```python
from build123d import *

# Parameters (mm, degrees)
SKETCH_1_W                    = 100
SKETCH_1_H                    = 80
EXTRUDE_1_DEPTH               = 19
SKETCH_2_W                    = 72
SKETCH_2_H                    = 92
CUT_EXTRUDE_1_DEPTH           = 17
SKETCH_3_W                    = 36.5
SKETCH_3_H                    = 54.5
EXTRUDE_2_DEPTH               = 17
SKETCH_4_W                    = 31.5
SKETCH_4_H                    = 49.5
CUT_EXTRUDE_2_DEPTH           = 17
HOLE_WIZARD_20_0_20_1_D       = 20
HOLE_WIZARD_20_0_20_1_DEPTH   = 2
HOLE_WIZARD_1_8_1_8_1_D       = 1.8
HOLE_WIZARD_1_8_1_8_2_D       = 1.8
HOLE_WIZARD_1_8_1_8_2_DEPTH   = 4
HOLE_WIZARD_1_8_1_8_3_D       = 1.8
HOLE_WIZARD_1_8_1_8_3_DEPTH   = 4
HOLE_WIZARD_2_35_2_35_1_D     = 2.35
HOLE_WIZARD_2_35_2_35_1_DEPTH = 2.5
HOLE_WIZARD_2_35_2_35_2_D     = 2.35
HOLE_WIZARD_2_35_2_35_2_DEPTH = 2.5
HOLE_WIZARD_2_35_2_35_3_D     = 2.35
HOLE_WIZARD_2_35_2_35_3_DEPTH = 2.5
HOLE_WIZARD_2_35_2_35_4_D     = 2.35
HOLE_WIZARD_2_35_2_35_4_DEPTH = 2.5
SKETCH_22_W                   = 13
SKETCH_22_H                   = 36.5
CUT_EXTRUDE_5_DEPTH           = 10
SKETCH_23_W                   = 80
SKETCH_23_H                   = 22.75
CUT_EXTRUDE_6_DEPTH           = 19
SKETCH_24_W                   = 17
SKETCH_24_H                   = 17.75
EXTRUDE_3_DEPTH               = 4
SKETCH_25_R                   = 0.9
EXTRUDE_4_DEPTH               = 4
EXTRUDE_START                 = -4
SKETCH_26_R                   = 0.9
EXTRUDE_5_DEPTH               = 4


with BuildPart() as part:
    # 스케치1 → 보스-돌출1 (new body)
    with BuildSketch(Plane(origin=(0, 0, 0), x_dir=(0, -1, 0), z_dir=(-1, 0, 0))):
        with Locations((-23.25, -14.25)):
            Rectangle(SKETCH_1_W, SKETCH_1_H)
    extrude(amount=-EXTRUDE_1_DEPTH)

    # 스케치2 → 컷-돌출1 (cut)
    with BuildSketch(Plane.ZY):
        with Locations((-14.25, 23.25)):
            Rectangle(SKETCH_2_W, SKETCH_2_H)
    extrude(amount=-CUT_EXTRUDE_1_DEPTH, mode=Mode.SUBTRACT)

    # 스케치3 → 보스-돌출2 (add)
    with BuildSketch(Plane.ZY.offset(-17)):
        with Locations((-14.25, 23.25)):
            Rectangle(SKETCH_3_W, SKETCH_3_H)
    extrude(amount=EXTRUDE_2_DEPTH)

    # 스케치4 → 컷-돌출2 (cut)
    with BuildSketch(Plane.ZY):
        with Locations((-14.25, 23.25)):
            Rectangle(SKETCH_4_W, SKETCH_4_H)
    extrude(amount=-CUT_EXTRUDE_2_DEPTH, mode=Mode.SUBTRACT)

    # Ø20.0 (20) 지름 구멍1
    with Locations(Plane.ZY.offset(-17)):
        with Locations((-14.25, 35.25)):
            Hole(HOLE_WIZARD_20_0_20_1_D / 2, depth=HOLE_WIZARD_20_0_20_1_DEPTH)

    # Ø1.8 (1.8) 지름 구멍1 (through all)
    with Locations(Plane.ZY):
        with Locations((-52.25, 71.25), (-14.25, 71.25), (23.75, 71.25), (23.75, -24.75), (-14.25, -24.75), (-52.25, -24.75), (-52.25, 23.25), (23.75, 23.25)):
            Hole(HOLE_WIZARD_1_8_1_8_1_D / 2)

    # Ø1.8 (1.8) 지름 구멍2
    with Locations(Plane.XY.offset(-50.25)):
        with Locations((12.975, -0.75), (12.975, 47.25)):
            Hole(HOLE_WIZARD_1_8_1_8_2_D / 2, depth=HOLE_WIZARD_1_8_1_8_2_DEPTH)

    # Ø1.8 (1.8) 지름 구멍3
    with Locations(Plane(origin=(0, 0, 21.75), x_dir=(-1, 0, 0), z_dir=(0, 0, -1))):
        with Locations((-12.975, -0.75), (-12.975, 47.25)):
            Hole(HOLE_WIZARD_1_8_1_8_3_D / 2, depth=HOLE_WIZARD_1_8_1_8_3_DEPTH)

    # Ø2.35 (2.35) 지름 구멍1
    with Locations(Plane(origin=(0, -1.5, 0), x_dir=(1, 0, 0), z_dir=(0, 1, 0))):
        with Locations((6, 6.25), (6, 22.25)):
            Hole(HOLE_WIZARD_2_35_2_35_1_D / 2, depth=HOLE_WIZARD_2_35_2_35_1_DEPTH)

    # Ø2.35 (2.35) 지름 구멍2
    with Locations(Plane.XY.offset(-30)):
        with Locations((6, 27.25), (6, 3.25)):
            Hole(HOLE_WIZARD_2_35_2_35_2_D / 2, depth=HOLE_WIZARD_2_35_2_35_2_DEPTH)

    # Ø2.35 (2.35) 지름 구멍3
    with Locations(Plane(origin=(0, 48, 0), x_dir=(-1, 0, 0), z_dir=(0, -1, 0))):
        with Locations((-6, 6.25), (-6, 22.25)):
            Hole(HOLE_WIZARD_2_35_2_35_3_D / 2, depth=HOLE_WIZARD_2_35_2_35_3_DEPTH)

    # Ø2.35 (2.35) 지름 구멍4
    with Locations(Plane(origin=(0, 0, 1.5), x_dir=(-1, 0, 0), z_dir=(0, 0, -1))):
        with Locations((-6, 27.25), (-6, 3.25)):
            Hole(HOLE_WIZARD_2_35_2_35_4_D / 2, depth=HOLE_WIZARD_2_35_2_35_4_DEPTH)

    # 스케치22 → 컷-돌출5 (cut)
    with BuildSketch(Plane.XZ.offset(26.75)):
        with Locations((6.5, -14.25)):
            Rectangle(SKETCH_22_W, SKETCH_22_H)
    extrude(amount=-CUT_EXTRUDE_5_DEPTH, mode=Mode.SUBTRACT)

    # 스케치23 → 컷-돌출6 (cut)
    with BuildSketch(Plane.ZY):
        with Locations((-14.25, 61.875)):
            Rectangle(SKETCH_23_W, SKETCH_23_H)
    extrude(amount=-CUT_EXTRUDE_6_DEPTH, mode=Mode.SUBTRACT)

    # 스케치24 → 보스-돌출3 (add)
    with BuildSketch(Plane(origin=(0, 50.5, 0), x_dir=(1, 0, 0), z_dir=(0, 1, 0))):
        with Locations((8.5, -12.875)):
            Rectangle(SKETCH_24_W, SKETCH_24_H)
        with Locations((8.5, 41.375)):
            Rectangle(SKETCH_24_W, SKETCH_24_H)
    extrude(amount=-EXTRUDE_3_DEPTH)

    # 스케치25 → 보스-돌출4 (add)
    with BuildSketch(Plane.XY.offset(25.75)):
        with Locations((12.975, 47.25)):
            Circle(SKETCH_25_R)
    extrude(amount=-EXTRUDE_4_DEPTH)

    # 스케치26 → 보스-돌출5 (add)
    with BuildSketch(Plane(origin=(0, 0, -54.25), x_dir=(-1, 0, 0), z_dir=(0, 0, -1)).offset(EXTRUDE_START)):
        with Locations((-12.975, 47.25)):
            Circle(SKETCH_26_R)
    extrude(amount=EXTRUDE_5_DEPTH)


solid = part.part
```
The model under review builds one solid part; all positions refer to its coordinate system, in mm. A direction names the side the tool comes from. Coordinates: 2 decimals unless noted, no trailing zeros. Write each loop counter-clockwise with the first axis right and the second up, starting at its lowest first coordinate (ties: lowest second). Pieces come first, ordered by that corner, then holes. Notation, with made-up numbers: (47.25, -30) -> (104.25, -30) arc R24 ccw to (104.25, 4) -> close; hole circle Ø7 at (54.25, 79.25). An arc over 180 degrees is marked (long way). One line per item, written item: value. Start each with the question number.
Q1. The part is to be moulded in two halves that separate along X. For faces 4 (the face through (6.153, -2.768, -23.415)), 5 (the face through (9.63, 23.86, -51.59)), 6 (the face through (19, 12, -14)), say which applies: +X half, -X half, draft (parallel to the pull), parting line (faces both ways), or undercut.
Q2. Clearance check with flat-ended pins moving along their axes: P1, Ø25, axis at y = 35, z = -17, coming from the -X side; P2, Ø2, axis at y = -24.75, z = -52.25, coming from the +X side; P3, Ø2, axis at x = 2.5, z = -16.5, coming from the -Y side; P4, Ø1.1, axis at x = 12.975, y = -0.75, coming from the -Z side. State where each tip first meets the part, or that it passes through.
Q3. Add section D-D, the plane y = 27.25. Give the boundary of the cut face in (x, z) (3 decimals).
Q4. Add section B-B, the plane y = 3.25. Give the boundary of the cut face in (x, z) (3 decimals), then the cut area to 3 significant figures.
Q5. To check wall thickness, follow probe 1 along Z at (x, y) = (6, 48.75) (3 decimals); probe 2 along Y at (x, z) = (13.5, 23.75); probe 3 along Z at (x, y) = (7, 17). State the ranges of each line that lie inside material, in increasing order.
Q6. Add section C-C, the plane x = 9.75. Give the boundary of the cut face in (y, z), then the cut area to 3 significant figures.
Q7. For faces 1 (the face through (6, -25, 4)), 2 (the face through (8, -1.5, -14)), 3 (the face through (5.847, 28.415, 2.768)), list the 3-axis set-ups (+Z, -Z, +X, -X, +Y, -Y) from which the entire face can be reached by the end or side of a thin tool; tool diameter is ignored.
Q8. Add section A-A, the plane z = -6.25. Give the boundary of the cut face in (x, y) (3 decimals).
Response:
1. face 4: undercut
1. face 5: draft
1. face 6: +X half
2. P1: x = 17
2. P2: x = 19
2. P3: y = -4
2. P4: z = -32.5
3. outline: (0, -54.25) -> (19, -54.25) -> (19, -20.25) -> (17, -20.25) -> (17, -30) -> (7.175, -30) -> (7.175, -32.5) -> (17, -32.5) -> (17, -50.25) -> (0, -50.25) -> close; (0, -32.5) -> (4.825, -32.5) -> (4.825, -30) -> (0, -30) -> close; (0, 1.5) -> (4.825, 1.5) -> (4.825, 4) -> (0, 4) -> close; (0, 21.75) -> (17, 21.75) -> (17, 4) -> (7.175, 4) -> (7.175, 1.5) -> (17, 1.5) -> (17, -8.25) -> (19, -8.25) -> (19, 25.75) -> (0, 25.75) -> close
4. outline: (0, -54.25) -> (19, -54.25) -> (19, 25.75) -> (0, 25.75) -> (0, 21.75) -> (17, 21.75) -> (17, 4) -> (7.175, 4) -> (7.175, 1.5) -> (17, 1.5) -> (17, -30) -> (7.175, -30) -> (7.175, -32.5) -> (17, -32.5) -> (17, -50.25) -> (0, -50.25) -> close; (0, -32.5) -> (4.825, -32.5) -> (4.825, -30) -> (0, -30) -> close; (0, 1.5) -> (4.825, 1.5) -> (4.825, 4) -> (0, 4) -> close
4. area: 369 mm²
5. probe 1: -54.25 to -23.425, -21.075 to -7.425, -5.075 to 25.75
5. probe 2: -26.75 to -25.65, -23.85 to -1.48, -0.02 to 22.35, 24.15 to 50.5
5. probe 3: -54.25 to -50.25, -32.5 to -30, 1.5 to 4, 21.75 to 25.75
6. outline: (-26.75, -54.25) -> (50.5, -54.25) -> (50.5, 25.75) -> (-26.75, 25.75) -> (-26.75, 4) -> (-22.75, 4) -> (-22.75, 21.75) -> (46.5, 21.75) -> (46.5, 4) -> (-4, 4) -> (-4, -32.5) -> (46.5, -32.5) -> (46.5, -50.25) -> (-22.75, -50.25) -> (-22.75, -32.5) -> (-26.75, -32.5) -> close; hole circle Ø1.8 at (-24.75, -52.25); hole circle Ø1.8 at (-24.75, 23.75); hole (-1.5, -30) -> (48, -30) -> (48, 1.5) -> (-1.5, 1.5) -> close; hole circle Ø1.8 at (23.25, -52.25); hole circle Ø1.8 at (23.25, 23.75)
6. area: 1,320 mm²
7. face 1: -X, -Y
7. face 2: -X
7. face 3: none
8. outline: (0, -4) -> (4.825, -4) -> (4.825, -1.5) -> (0, -1.5) -> close; (0, 48) -> (4.825, 48) -> (4.825, 50.5) -> (0, 50.5) -> close; (7.175, -4) -> (17, -4) -> (17, -22.75) -> (13, -22.75) -> (13, -26.75) -> (19, -26.75) -> (19, 29.25) -> (17, 29.25) -> (17, -1.5) -> (7.175, -1.5) -> close; (7.175, 48) -> (17, 48) -> (17, 41.25) -> (19, 41.25) -> (19, 50.5) -> (7.175, 50.5) -> close
